```python
from build123d import *

# Parameters (mm, degrees)
SKETCH1_W           = 125
SKETCH1_H           = 8
SKETCH1_R           = 1.75
BOSS_EXTRUDE1_DEPTH = 5
CUT_EXTRUDE1_DEPTH  = 64.207990001
CHAMFER1_SIZE       = 2


with BuildPart() as part:
    # Sketch1 → Boss-Extrude1 (new body)
    with BuildSketch(Plane(origin=(0, 0, 0), x_dir=(0, 1, 0), z_dir=(0, 0, 1))):
        Rectangle(SKETCH1_W, SKETCH1_H)
        with Locations(Location((-56.5, 0, 0), (0, 0, 270))):
            Circle(SKETCH1_R, mode=Mode.SUBTRACT)
        with Locations(Location((56.5, 0, 0), (0, 0, 270))):
            Circle(SKETCH1_R, mode=Mode.SUBTRACT)
    extrude(amount=BOSS_EXTRUDE1_DEPTH)

    # Sketch2 → Cut-Extrude1 (cut, through all)
    with BuildSketch(Plane.YZ.offset(4)):
        Polygon((-40, 3), (-43, 0), (43, 0), (40, 3), align=None)
        Polygon((-60.5, 0), (-62.5, 5), (-62.5, 0), align=None)
        Polygon((62.5, 5), (60.5, 0), (62.5, 0), align=None)
    extrude(amount=-CUT_EXTRUDE1_DEPTH, mode=Mode.SUBTRACT)

    # Chamfer1
    chamfer1_edges = [part.edges().sort_by_distance(p)[0] for p in [
        (-1.75, -56.5, 0),
        (-1.75, 56.5, 0),
    ]]
    chamfer(chamfer1_edges, length=CHAMFER1_SIZE)


solid = part.part
```
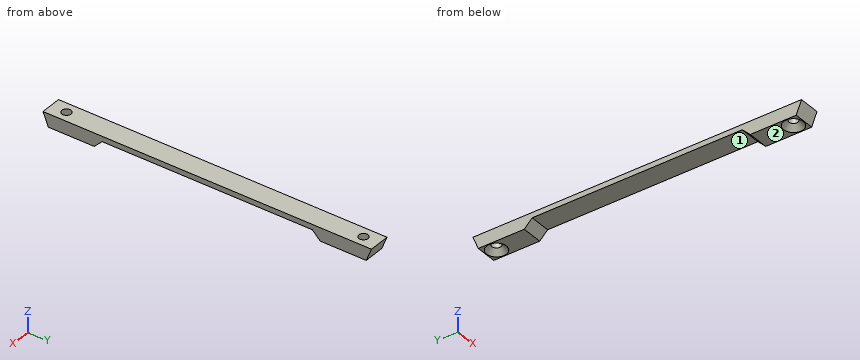
Can you work these out from the model? Positions are in its coordinate system, mm. Face numbers are marked on the shaded views. Coordinates: 2 decimals unless noted, no trailing zeros. Loops run counter-clockwise (first coordinate to the right, second up) from the corner with the lowest first, then second, coordinate; pieces in that order, holes last. Notation, with made-up numbers: (25, -3) - (65, -3) arc R7 cw to (65, 6) - close; hole circle Ø1 at (-35.75, -8). An arc over 180 degrees is marked (long way). Answer as CSV lines item,"result". Start each with the question number.
1) Thinking about a two-plate mould opening in Y: for the marked faces 1 and 2, which applies, pulls with the +Y half, pulls with the -Y half, needs draft (parallel to the pull), parting line crosses it, or undercut?
2) Suppose I cut it at D-D (y = 13). Please give me the cut outline in (x, z).
3) Suppose I cut it at C-C (z = 3.95). Please give me the cut outline in (x, y), plus the area to 3 significant figures.
4) Suppose I cut it at A-A (x = 0). Please give me the cut outline in (y, z).
5) I need wall thicknesses on line 1 (Y direction, x = -2, z = 0.7); line 2 (Y direction, x = 0, z = 3.6); line 3 (Y direction, x = 0, z = 2.85). Which ranges of each line are inside material? Lowest first, please. Write a range as from..to.
6) Suppose I cut it at B-B (y = -56.5). Please give me the cut outline in (x, z).
7) For pin 1 (2 mm diameter, centred on x = -2, z = 3.5, fed in from +Y); pin 2 (3 mm diameter, centred on x = 0, y = 56.5, fed in from -Z); pin 3 (1 mm diameter, centred on x = 2.5, z = 1, fed in from -Y), each with a flat end and sliding along its axis, tell me the tip position at first contact or that it passes through.
Check result:
1,face 1,"undercut"
1,face 2,"needs draft"
2,outline,"(-4, 3) - (4, 3) - (4, 5) - (-4, 5) - close"
3,outline,"(-4, -62.08) - (4, -62.08) - (4, 62.08) - (-4, 62.08) - close; hole circle Ø3.5 at (0, -56.5); hole circle Ø3.5 at (0, 56.5)"
3,area,"974 mm²"
4,outline,"(-62.5, 5) - (-60.5, 0) - (-60.25, 0) - (-58.25, 2) - (-58.25, 5) - close; (-54.75, 2) - (-52.75, 0) - (-43, 0) - (-40, 3) - (40, 3) - (43, 0) - (52.75, 0) - (54.75, 2) - (54.75, 5) - (-54.75, 5) - close; (58.25, 2) - (60.25, 0) - (60.5, 0) - (62.5, 5) - (58.25, 5) - close"
5,line 1,"y = -60.78..-58.8, -54.2..-42.3, 42.3..54.2, 58.8..60.78"
5,line 2,"y = -61.94..-58.25, -54.75..54.75, 58.25..61.94"
5,line 3,"y = -61.64..-58.25, -54.75..-40.15, 40.15..54.75, 58.25..61.64"
6,outline,"(-4, 0) - (-3.75, 0) - (-1.75, 2) - (-1.75, 5) - (-4, 5) - close; (1.75, 2) - (3.75, 0) - (4, 0) - (4, 5) - (1.75, 5) - close"
7,pin 1,"stops at y = 62.3"
7,pin 2,"passes through"
7,pin 3,"stops at y = -61.1"
